Autodesk Inventor part; units mm, degrees
ref_plane "YZ Plane" through (0, 0, 0) normal (1, 0, 0) x (0, 1, 0)
ref_plane "XZ Plane" through (0, 0, 0) normal (0, 1, 0) x (-1, 0, 0)
ref_plane "XY Plane" through (0, 0, 0) normal (0, 0, 1) x (1, 0, 0)
sketch "Sketch1" plane through (0, 0, 0) normal (0, 1, 0) x (-1, 0, 0)
  line L0 (15.24, 9.525) -> (-3.81, 9.525)
  line L1 (-3.81, 9.525) -> (-3.81, -9.525)
  line L2 (-3.81, -9.525) -> (15.24, -9.525)
  line L3 (15.24, -9.525) -> (15.24, 9.525)
  point P0 (0, 0)
  dimension "d0" = 19.05
  dimension "d1" = 19.05
extrude "Extrusion1" add sketch "Sketch1" along normal blind 25.4
sketch "Sketch2" plane through (0, 25.4, 0) normal (0, 1, 0) x (1, 0, 0)
  line L0 (-15.24, -9.525) -> (3.81, -9.525)
  line L1 (-5.715, -9.525) -> (-5.715, 9.525)
  line L2 (3.81, 9.525) -> (-15.24, 9.525)
  line L3 (-15.24, 9.525) -> (-15.24, -9.525)
  line L4 (-15.24, 0) -> (3.81, 0)
  line L5 (3.81, -9.525) -> (3.81, 9.525)
  point P0 (0, 0)
sketch "Sketch3" plane through (0, 25.4, 0) normal (0, 1, 0) x (1, 0, 0)
  circle A0 centre (-5.715, 0) radius 4.8895 construction
  line L0 (3.81, -9.525) -> (3.81, 9.525) construction
  line L1 (3.81, 9.525) -> (-15.24, 9.525) construction
  circle A1 centre (-5.715, 0) radius 4.8895
  point P0 (0, 0)
  dimension "d4" = 9.779
  dimension "d5" = 9.525
  dimension "d6" = 9.525
extrude "Extrusion2" cut sketch "Sketch3" against normal through all
sketch "Sketch4" plane through (3.81, 0, 9.525) normal (1, 0, 0) x (0, 0, -1)
  circle A0 centre (9.525, 12.7) radius 1.3176
  line L0 (19.05, 0) -> (19.05, 25.4)
  line L1 (0, 25.4) -> (19.05, 25.4)
  point P0 (9.525, 0)
  dimension "d9" = 2.6353
  dimension "d10" = 9.525
  dimension "d11" = 12.7
extrude "Extrusion3" cut sketch "Sketch4" against normal through all
properties part number "drill holder"
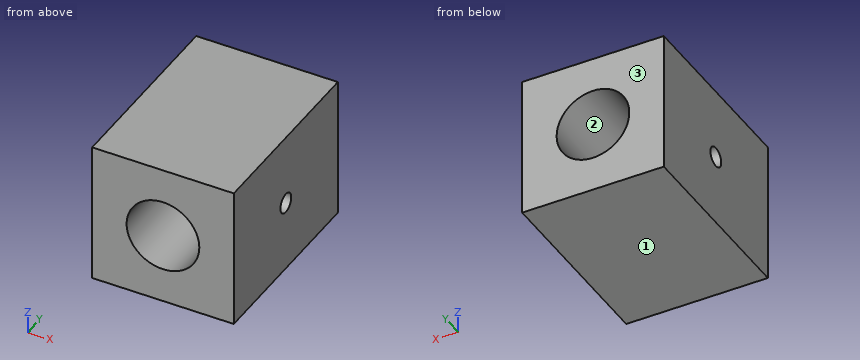
Can you work these out from the model? Positions are in its coordinate system, mm. Face numbers are marked on the shaded views. Coordinates: 2 decimals unless noted, no trailing zeros. Loops run counter-clockwise (first coordinate to the right, second up) from the corner with the lowest first, then second, coordinate; pieces in that order, holes last. Notation, with made-up numbers: (-12.5, -21) - (-8.5, -21) arc R19 ccw to (-8.5, 7) - close; hole circle Ø3 at (70, 2). An arc over 180 degrees is marked (long way). Put each result on its own line as item: value. Start each with the question number.
Item 1: If I drill on line 1 along Z through (x, y) = (1.4, 12.7) (3 decimals); line 2 along X through (y, z) = (19, 0); line 3 along Y through (x, z) = (-13.4, 0), over which ranges is the centre line in solid material (lowest first)?
Item 2: Suppose I cut it at D-D (y = 6). Please give me the cut outline in (x, z) (1 decimal), and give its area (3 significant figures).
Item 3: Suppose I cut it at A-A (z = 0). Please give me the cut outline in (x, y).
Item 4: Suppose I cut it at B-B (y = 12.7). Please give me the cut outline in (x, z) (1 decimal), and give its area (3 significant figures).
Item 5: For pin 1 (1 mm diameter, centred on x = -5.5, z = 2.5, fed in from -Y), with a flat end and sliding along its axis, tell me the tip position at first contact or that it passes through.
Item 6: If we mould it in two halves opening along Z, with no side actions, what happens to the marked faces 1, 2 and 3? For each: +Z half, -Z half, draft (parallel to the pull), parting line (faces both ways), or undercut.
Item 7: Suppose I cut it at C-C (x = -6.75). Please give me the cut outline in (y, z) (3 decimals), and give its area (3 significant figures).
Here are the results:
1. line 1: -9.525 to -1.318, 1.318 to 9.525
1. line 2: -15.24 to -10.6, -0.83 to 3.81
1. line 3: 0 to 11.38, 14.02 to 25.4
2. outline: (-15.2, -9.5) - (3.8, -9.5) - (3.8, 9.5) - (-15.2, 9.5) - close; hole circle Ø9.8 at (-5.7, 0)
2. area: 288 mm²
3. outline: (-15.24, 0) - (-10.6, 0) - (-10.6, 11.38) - (-15.24, 11.38) - close; (-15.24, 14.02) - (-10.6, 14.02) - (-10.6, 25.4) - (-15.24, 25.4) - close; (-0.83, 0) - (3.81, 0) - (3.81, 11.38) - (-0.83, 11.38) - close; (-0.83, 14.02) - (3.81, 14.02) - (3.81, 25.4) - (-0.83, 25.4) - close
4. outline: (-15.2, -9.5) - (3.8, -9.5) - (3.8, -1.3) - (-1, -1.3) arc R4.9 cw to (-10.4, -1.3) - (-15.2, -1.3) - close; (-15.2, 1.3) - (-10.4, 1.3) arc R4.9 cw to (-1, 1.3) - (3.8, 1.3) - (3.8, 9.5) - (-15.2, 9.5) - close
4. area: 263 mm²
5. pin 1: through
6. face 1: -Z half
6. face 2: undercut
6. face 3: draft
7. outline: (0, -9.525) - (25.4, -9.525) - (25.4, -4.779) - (0, -4.779) - close; (0, 4.779) - (25.4, 4.779) - (25.4, 9.525) - (0, 9.525) - close
7. area: 241 mm²
